from build123d import *

# Parameters (mm, degrees)
F0_W     = 25.4
F0_H     = 50.8
F0_W_2   = 20.32
F0_H_2   = 45.72
F1_DEPTH = 146.05
F2_R     = 2.5527
F3_DEPTH = 76.2
F4_R     = 14.2875
F5_DEPTH = 25.4


# Not quite as in the source:
# - a feature names something its author has since deleted; it is built from what else it names


with BuildPart() as f1:
    # F0 (on Top) → F1 (new body)
    with BuildSketch(Plane.XY):
        with Locations((12.7, -25.4)):
            Rectangle(F0_W, F0_H)
        with Locations((12.7, -25.4)):
            Rectangle(F0_W_2, F0_H_2, mode=Mode.SUBTRACT)
    extrude(amount=F1_DEPTH)

    # F2 (on face) → F3 (cut)
    with BuildSketch(Plane.XZ.offset(50.8)):
        with Locations((12.7, 88.9)):
            Circle(F2_R)
        with Locations((12.7, 63.5)):
            Circle(F2_R)
        with Locations((12.7, 38.1)):
            Circle(F2_R)
        with Locations((12.7, 12.7)):
            Circle(F2_R)
        with Locations((12.7, 114.3)):
            Circle(F2_R)
        with Locations((12.7, 139.7)):
            Circle(F2_R)
    extrude(amount=-F3_DEPTH, mode=Mode.SUBTRACT)

    # F4 (on face) → F5 (cut)
    with BuildSketch(Plane.YZ.offset(25.4)):
        with Locations((-25.4, 120.65)):
            Circle(F4_R)
        with BuildLine():
            ThreePointArc((-50.8, 120.65), (-43.3605122421, 138.6105122421), (-25.4, 146.05))
            Line((-25.4, 146.05), (-50.8, 146.05))
            Line((-50.8, 146.05), (-50.8, 120.65))
        make_face()
        with BuildLine():
            ThreePointArc((-25.4, 146.05), (-7.4394877579, 138.6105122421), (0, 120.65))
            Line((0, 120.65), (0, 146.05))
            Line((0, 146.05), (-25.4, 146.05))
        make_face()
    extrude(amount=-F5_DEPTH, mode=Mode.SUBTRACT)


solid = f1.part
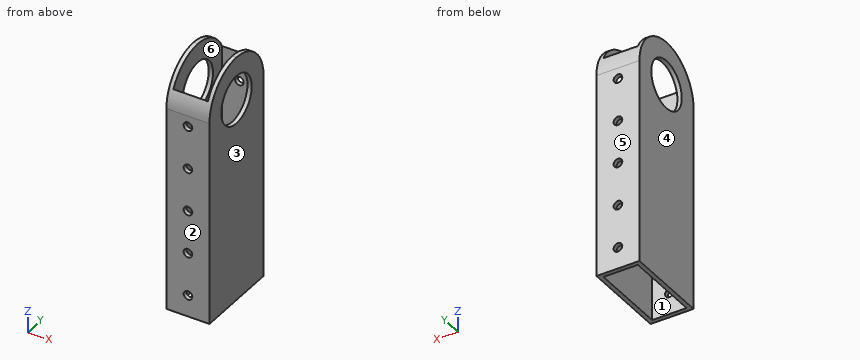
The model under review builds one solid part; all positions refer to its coordinate system, in mm. Face numbers are marked on the shaded views. A direction names the side the tool comes from. Round coordinates to 2 decimals unless told otherwise and drop trailing zeros. Loops run counter-clockwise (first coordinate to the right, second up) from the corner with the lowest first, then second, coordinate; pieces in that order, holes last. Notation, with made-up numbers: (4.25, 82.5) -> (11.25, 82.5) arc R24 ccw to (11.25, 94.5) -> close; hole circle Ø7 at (75.25, 19.5). An arc over 180 degrees is marked (long way). Answer as CSV lines item,"result".
1) Add section B-B on z = 38.1. Write out the cut boundary in (x, y), plus the area to 3 significant figures.
Geometry results:
outline,"(0, -50.8) -> (10.15, -50.8) -> (10.15, -48.26) -> (2.54, -48.26) -> (2.54, -2.54) -> (10.15, -2.54) -> (10.15, 0) -> (0, 0) -> close; (15.25, -50.8) -> (25.4, -50.8) -> (25.4, 0) -> (15.25, 0) -> (15.25, -2.54) -> (22.86, -2.54) -> (22.86, -48.26) -> (15.25, -48.26) -> close"
area,"335 mm²"
2) Draft analysis for pull direction X (two halves, no side actions). For the marked faces 3, 4, 5 and 6, state which applies: pulls with the +X half, pulls with the -X half, needs draft (parallel to the pull), parting line crosses it, or undercut.
Geometry results:
face 3,"pulls with the +X half"
face 4,"pulls with the -X half"
face 5,"needs draft"
face 6,"undercut"
3) Tool access review of the marked faces 1 and 2: name each direction out of +Z, -Z, +X, -X, +Y, -Y from which nothing blocks a thin tool from reaching the whole face with its end or side.
Geometry results:
face 1,"+Z, -Z"
face 2,"+Z, -Z, +X, -X, -Y"
4) To check wall thickness, follow line 1 along Z through (x, y) = (2.25, -26); line 2 along Y through (x, z) = (20.5, 90); line 3 along X through (y, z) = (-23.5, 46). State the ranges of each line that lie inside material, in increasing order. Write a range as from..to.
Geometry results:
line 1,"z = 0..106.38, 134.92..146.04"
line 2,"y = -50.8..-48.26, -2.54..0"
line 3,"x = 0..2.54, 22.86..25.4"
5) For P1, Ø4, axis at x = 12.7, z = 88.9, coming from the +Y side, flat-tipped, find the tip position at first contact; note if it passes through.
Geometry results:
P1,"passes through"
6) Add section A-A on x = 18.5. Write out the cut boundary in (y, z), plus the area to 3 significant figures.
Geometry results:
outline,"(-50.8, 0) -> (-48.26, 0) -> (-48.26, 131.72) arc R25.4 ccw to (-50.8, 120.65) -> close; (-2.54, 0) -> (0, 0) -> (0, 120.65) arc R25.4 ccw to (-2.54, 131.72) -> close"
area,"651 mm²"
7) Add section C-C on y = -36. Write out the cut boundary in (x, z), plus the area to 3 significant figures.
Geometry results:
outline,"(0, 0) -> (2.54, 0) -> (2.54, 111.07) -> (0, 111.07) -> close; (0, 130.23) -> (2.54, 130.23) -> (2.54, 143.73) -> (0, 143.73) -> close; (22.86, 0) -> (25.4, 0) -> (25.4, 111.07) -> (22.86, 111.07) -> close; (22.86, 130.23) -> (25.4, 130.23) -> (25.4, 143.73) -> (22.86, 143.73) -> close"
area,"633 mm²"
8) Add section D-D on z = 114.3. Write out the cut boundary in (x, y).
Geometry results:
outline,"(0, -50.8) -> (10.15, -50.8) -> (10.15, -48.26) -> (2.54, -48.26) -> (2.54, -38.2) -> (0, -38.2) -> close; (0, -12.6) -> (2.54, -12.6) -> (2.54, -2.54) -> (10.15, -2.54) -> (10.15, 0) -> (0, 0) -> close; (15.25, -50.8) -> (25.4, -50.8) -> (25.4, -38.2) -> (22.86, -38.2) -> (22.86, -48.26) -> (15.25, -48.26) -> close; (15.25, -2.54) -> (22.86, -2.54) -> (22.86, -12.6) -> (25.4, -12.6) -> (25.4, 0) -> (15.25, 0) -> close"
